from build123d import *

# Parameters (mm, degrees)
SKETCH1_R           = 5.164999999999999
SKETCH1_R_2         = 2.675
BOSS_EXTRUDE1_DEPTH = 6
CHAMFER1_SIZE       = 6
CHAMFER1_SIZE_2     = 1.77728097
CUT_EXTRUDE1_DEPTH  = 10.452748277617466
BOSS_EXTRUDE2_START = 0.5
BOSS_EXTRUDE2_DEPTH = 0.5
FILLET1_R           = 0.5


with BuildPart() as part:
    # Sketch1 → Boss-Extrude1 (new body)
    with BuildSketch(Plane(origin=(0, 0, 0), x_dir=(1, 0, 0), z_dir=(0, 1, 0))):
        with Locations(Location((0, 0, 0), (0, 0, 270))):
            Circle(SKETCH1_R)
        with Locations(Location((0, 0, 0), (0, 0, 270))):
            Circle(SKETCH1_R_2, mode=Mode.SUBTRACT)
    extrude(amount=BOSS_EXTRUDE1_DEPTH)

    # Chamfer1
    # the kernel refuses this chamfer: 6, 1.77728097 mm, written as the material it takes off along each edge
    with BuildSketch(Plane(origin=(0, 6, 0), x_dir=(-1.8e-16, 0, 1), z_dir=(-1, 0, -1.8e-16))) as chamfer1_piece_1:
        Polygon((5.164999999999999, -CHAMFER1_SIZE), (5.164999999999999 - CHAMFER1_SIZE_2, 0), (5.164999999999999, 0), align=None)
    revolve(axis=Axis((0, 6, 0), (0, 1, 0)), mode=Mode.SUBTRACT)

    # Sketch2 → Cut-Extrude1 (cut, through all)
    with BuildSketch(Plane(origin=(0, 6, 0), x_dir=(1, 0, 0), z_dir=(0, 1, 0))):
        Polygon((-6e-17, 0.5), (-6.017243985575578, 0.4999999999999993), (-6.017243985575578, -0.5000000000000008), (6e-17, -0.5), align=None)
    extrude(amount=-CUT_EXTRUDE1_DEPTH, mode=Mode.SUBTRACT)

    # Sketch3 → Boss-Extrude2 (add)
    with BuildSketch(Plane.XZ.offset(BOSS_EXTRUDE2_START)):
        with BuildLine():
            Line((-2.6278555896395814, -0.4999999999999993), (-5.140741678007149, -0.49999999999999917))
            ThreePointArc((-5.140741678007149, -0.49999999999999917), (5.164999999999977, -2.29e-15), (-5.140741678007172, 0.5000000000000027))
            Line((-5.140741678007172, 0.5000000000000027), (-2.627855589639582, 0.5000000000000001))
            ThreePointArc((-2.627855589639582, 0.5000000000000001), (2.6749999999999985, 0), (-2.6278555896395814, -0.4999999999999993))
        make_face()
    extrude(amount=-BOSS_EXTRUDE2_DEPTH)

    # Fillet1
    fillet1_edges = [part.edges().sort_by_distance(p)[0] for p in [
        (2.6750000000000003, 6, -1.288e-14),
        (2.674999999999999, -0.5, 5.4e-16),
    ]]
    fillet(fillet1_edges, radius=FILLET1_R)


solid = part.part
Design review of the part built by this model. Coordinates are the model's own, in mm. A direction names the side the tool comes from. Coordinates: 2 decimals unless noted, no trailing zeros. Write each loop counter-clockwise with the first axis right and the second up, starting at its lowest first coordinate (ties: lowest second). Pieces come first, ordered by that corner, then holes. Notation, with made-up numbers: (-11.5, 5.25) - (-5.5, 5.25) arc R22 ccw to (-5.5, 27.25) - close; hole circle Ø6 at (-21.75, 20). An arc over 180 degrees is marked (long way). Use one line per item in the form item = value.
Q1. Insertion check: pin 1 Ø4.5 at (x, z) = (0, 0) entering from +Y; pin 2 Ø5 at (x, z) = (-0.5, 3) entering from +Y; pin 3 Ø0.8 at (x, y) = (-4, 2.5) entering from -Z; pin 4 Ø1.3 at (x, y) = (-4, 2.5) entering from +Z. Each pin has a flat end and moves straight along its axis. Give the tip position at first contact, or say it passes through.
Taken from the geometry:
pin_1 = through
pin_2 = 6
pin_3 = -2.61
pin_4 = 2.95
Q2. Consider section D-D (y = 5.25). Write out the cut boundary in (x, z) (3 decimals), plus the area to 3 significant figures.
Taken from the geometry:
outline = (-3.575, -0.5) arc R3.61 ccw (long way) to (-3.575, 0.5) - (-2.628, 0.5) arc R2.675 cw (long way) to (-2.628, -0.5) - close
area = 17.5 mm^2
Q3. Consider section A-A (z = 0). Write out the cut boundary in (x, y) (3 decimals), plus the area to 3 significant figures.
Taken from the geometry:
outline = (2.675, 0) arc R0.5 ccw to (3.175, -0.5) - (5.165, -0.5) - (5.165, 0) - (3.388, 6) - (3.175, 6) arc R0.5 ccw to (2.675, 5.5) - close
area = 10.7 mm^2
Q4. Machinability: for faces 4 (the cylindrical face through (2.673, 2.712, 0.111)), 5 (the flat face through (-4, 2, 0.5)), which of the approach directions +Z, -Z, +X, -X, +Y, -Y give a long, thin tool a straight path to every point of the face, cutting with its end or side? Answer none if there is none.
Taken from the geometry:
face_4 = +Y, -Y
face_5 = -X, +Y, -Y
Q5. For probe 1 along Z at (x, y) = (-4, 2); probe 2 along Z at (x, y) = (0, 1.2) (3 decimals); probe 3 along X at (y, z) = (2.25, -3.5), list the stretches that pass through material, from the lowest coordinate up.
Taken from the geometry:
probe_1 = -2.22 to -0.5, 0.5 to 2.22
probe_2 = -4.81 to -2.675, 2.675 to 4.81
probe_3 = -2.83 to 2.83
Q6. Consider section B-B (x = 0). Write out the cut boundary in (y, z) (3 decimals).
Taken from the geometry:
outline = (-0.5, -5.165) - (0, -5.165) - (6, -3.388) - (6, -3.175) arc R0.5 ccw to (5.5, -2.675) - (0, -2.675) arc R0.5 ccw to (-0.5, -3.175) - close; (-0.5, 3.175) arc R0.5 ccw to (0, 2.675) - (5.5, 2.675) arc R0.5 ccw to (6, 3.175) - (6, 3.388) - (0, 5.165) - (-0.5, 5.165) - close
Q7. Consider section C-C (y = 4.5). Write out the cut boundary in (x, z) (3 decimals), plus the area to 3 significant figures.
Taken from the geometry:
outline = (-3.799, -0.5) arc R3.832 ccw (long way) to (-3.799, 0.5) - (-2.628, 0.5) arc R2.675 cw (long way) to (-2.628, -0.5) - close
area = 22.5 mm^2
Q8. The part is to be moulded in two halves that separate along Z. For faces 1 (the cylindrical face through (5.16, -0.25, -0.22)), 2 (the flat face through (-4, 2, -0.5)), 3 (the flat face through (3.4, -0.5, 0.1)), say which applies: +Z half, -Z half, draft (parallel to the pull), parting line (faces both ways), or undercut.
Taken from the geometry:
face_1 = parting line
face_2 = undercut
face_3 = draft
